Here's how the part is built. I have some questions about the finished solid (model axes, mm). A direction names the side the tool comes from. Round coordinates to 2 decimals unless told otherwise and drop trailing zeros. Order: outer loops, then holes, each group sorted by start corner. A loop starts at its lowest first (then second) coordinate and runs counter-clockwise, first axis right, second up.
Autodesk Inventor part; units mm, degrees
ref_plane "YZ Plane" through (0, 0, 0) normal (1, 0, 0) x (0, 1, 0)
ref_plane "XZ Plane" through (0, 0, 0) normal (0, 1, 0) x (-1, 0, 0)
ref_plane "XY Plane" through (0, 0, 0) normal (0, 0, 1) x (1, 0, 0)
sketch "Sketch1" plane through (0, 0, 0) normal (0, 0, 1) x (1, 0, 0)
  line L0 (0, 40.85) -> (0, 0)
  line L1 (0, 0) -> (-17, 0)
  line L2 (-17, 0) -> (-17, -5)
  line L3 (-17, -5) -> (5, -5)
  line L4 (5, -5) -> (5, 40.85)
  line L5 (5, 40.85) -> (0, 40.85)
  line L6 (-17, 0) -> (-17, 4)
  line L7 (-17, 4) -> (-15, 4)
  line L8 (-15, 4) -> (-15, 0)
  line L9 (-17, -5) -> (-17, -9)
  line L10 (-17, -9) -> (-15, -9)
  line L11 (-15, -9) -> (-15, -5)
  line L12 (-9, 0) -> (-9, 4)
  line L13 (-9, 4) -> (0, 4)
  line L14 (-9, -5) -> (-9, -9)
  line L15 (-9, -9) -> (5, -9)
  line L16 (5, -9) -> (5, -5)
  line L17 (-15, 4) -> (-9, 4)
  line L18 (-15, -9) -> (-9, -9)
  dimension "d0" = 5
  dimension "d1" = 15
  dimension "d2" = 4
  dimension "d3" = 2
  dimension "d4" = 40.85
  dimension "d5" = 6
extrude "Extrusion1" add sketch "Sketch1" along normal blind 25
sketch "Sketch2" plane through (-17, 4, 0) normal (0, 1, 0) x (1, 0, 0)
  circle A0 centre (-1.4373, -213.5) radius 4.5
  line L0 (16.4159, -222.1385) -> (44.0445, -254.6126)
  line L1 (44.0445, -254.6126) -> (38.713, -259.1485)
  line L2 (38.713, -259.1485) -> (11.0845, -226.6745)
  line L3 (11.0845, -226.6745) -> (16.4159, -222.1385)
  line L4 (1.9901, -210.584) -> (-347.6847, 200.416)
  circle A1 centre (-351.112, 197.5) radius 4.5
  point P0 (17, 0)
  point P1 (41.3788, -256.8805)
  dimension "d8" = 7
extrude "Extrusion2" cut sketch "Sketch2" against normal blind 3 contours L0 L1 L2 L3
sketch "Sketch3" plane through (-17, -9, 0) normal (0, -1, 0) x (1, 0, 0)
  line L0 (1.9991, 25) -> (2.3222, 0)
  line L1 (9.3228, 0) -> (8.9997, 25)
  line L2 (22, 225.4393) -> (22, 219.5607) construction
  line L3 (22, 225.4393) -> (-378, 225.4393) construction
  line L4 (-378, 219.5607) -> (-378, 225.4393) construction
  line L5 (22, 219.5607) -> (-378, 219.5607) construction
  circle A0 centre (6.5, 222.5) radius 4.5 construction
  line L6 (-355.6868, -191.4906) -> (9.8625, 219.5094) construction
  line L7 (70.9842, 282.9643) -> (65.7537, 287.6164)
  line L8 (65.7537, 287.6164) -> (-8.4745, 204.1589)
  line L9 (-8.4745, 204.1589) -> (-3.244, 199.5068)
  line L10 (-3.244, 199.5068) -> (70.9842, 282.9643)
  line L11 (2.3222, 0) -> (9.3228, 0)
  line L12 (8.9997, 25) -> (1.9991, 25)
  circle A1 centre (-359.0493, -188.5) radius 4.5
  point P0 (17, 0)
  point P1 (68.369, 285.2903)
  dimension "d38" = 7
extrude "Extrusion3" cut sketch "Sketch3" against normal blind 3 contours L10 L9 L8 L7
chamfer "Chamfer1" distance 7.75 angle 45 1 edges at (5, -9, 12.5)
chamfer "Chamfer3" distance 6 angle 45 1 edges at (0, 4, 12.5)
sketch "Sketch5" plane through (0, 40.85, 0) normal (-1, 0, 0) x (0, 0, 1)
  line L0 (212.5, -7.0607) -> (212.5, -12.9393)
  line L1 (-187.5, -7.0607) -> (212.5, -7.0607)
  line L2 (-187.5, -12.9393) -> (-187.5, -7.0607)
  line L3 (-187.5, -12.9393) -> (212.5, -12.9393)
  line L4 (12.5, -7.0607) -> (12.5, -12.9393) construction
  line L5 (12.5, -10) -> (25, -10) construction
  line L6 (25, -42.1) -> (25, 0)
  line L7 (12.5, -10) -> (0, -10) construction
  line L8 (0, -42.1) -> (0, 0)
  point P0 (0, -40.85)
hole "Hole1" at (0, 30.85, 12.5) direction (1, 0, 0) diameter 3.4 end through all counterbore diameter 6.5 counterbore depth 3.4
fillet "Fillet3" radius 2 6 edges at (-17, 4, 12.5) (-17, -9, 12.5) (5, -1.25, 12.5) (0, 10, 12.5) (5, 40.85, 12.5) (0, 40.85, 12.5)
chamfer "Chamfer4" [suppressed]
properties part number "belt no touchy"
1. If we section it at B-B, the plane z = 12.5: Write out the boundary of the cut face in (x, y).
Evaluation:
outline: (-17, -7) arc R2 ccw to (-15, -9) - (-2.75, -9) - (4.41, -1.84) arc R2 ccw to (5, -0.42) - (5, 29.15) - (3.4, 29.15) - (3.4, 27.6) - (0, 27.6) - (0, 10.83) arc R2 cw to (-0.59, 9.41) - (-6, 4) - (-15, 4) arc R2 ccw to (-17, 2) - close; (0, 34.1) - (3.4, 34.1) - (3.4, 32.55) - (5, 32.55) - (5, 38.85) arc R2 ccw to (3, 40.85) - (2, 40.85) arc R2 ccw to (0, 38.85) - close
2. I'm going to push flat-ended pins straight in: P1, Ø4, axis at y = 23.5, z = 21, coming from the -X side; P2, Ø2.5, axis at x = -12, z = 9, coming from the +Y side; P3, Ø5, axis at x = 1.5, z = 5, coming from the -Y side. Where does each tip first touch, or does it pass through?
Evaluation:
P1: stops at x = 0
P2: stops at y = 4
P3: stops at y = -7.25
3. If we mould it in two halves opening along Z, with no side actions, what happens to faces 4 (the cylindrical face through (-16.43, -8.4, 12.68)), 5 (the flat face through (-4, 5, 0)), 6 (the flat face through (3.4, 32, 14))? For each: released by +Z, released by -Z, zero draft, split by the parting line, or undercut.
Evaluation:
face 4: zero draft
face 5: released by -Z
face 6: undercut
4. If we section it at A-A, the plane y = 30.85: Write out the boundary of the cut face in (x, z).
Evaluation:
outline: (0, 0) - (5, 0) - (5, 10.8) - (3.4, 10.8) - (3.4, 9.25) - (0, 9.25) - close; (0, 15.75) - (3.4, 15.75) - (3.4, 14.2) - (5, 14.2) - (5, 25) - (0, 25) - close
5. If we section it at D-D, the plane x = -5.5: Write out the boundary of the cut face in (y, z).
Evaluation:
outline: (-9, 0) - (4.5, 0) - (4.5, 25) - (-9, 25) - close
6. On a 3-axis mill with a long thin cutter (end or side, diameter ignored), from which of +Z, -Z, +X, -X, +Y, -Y can I reach the whole of each face in a straight line? I mean faces 1 (the cylindrical face through (4.21, 32.36, 13.28)), 2 (the flat face through (0, 25, 12)), 3 (the cylindrical face through (1.7, 32.8, 9.9)). Say none if no direction works.
Evaluation:
face 1: +X, -X
face 2: +Z, -Z, -X, +Y
face 3: -X
7. If we section it at C-C, the plane z = 19.25: Write out the boundary of the cut face in (x, y), and give its area (3 significant figures).
Evaluation:
outline: (-17, -7) arc R2 ccw to (-15, -9) - (-2.75, -9) - (4.41, -1.84) arc R2 ccw to (5, -0.42) - (5, 38.85) arc R2 ccw to (3, 40.85) - (2, 40.85) arc R2 ccw to (0, 38.85) - (0, 10.83) arc R2 cw to (-0.59, 9.41) - (-6, 4) - (-15, 4) arc R2 ccw to (-17, 2) - close
area: 455 mm2
8. I need wall thicknesses on probe 1 along Z at (x, y) = (4.2, 30.85); probe 2 along Z at (x, y) = (1.75, 30.85); probe 3 along Y at (x, z) = (-6.75, 3). Which ranges of each line are inside material? Lowest first, please.
Evaluation:
probe 1: z = 0 to 10.8, 14.2 to 25
probe 2: z = 0 to 9.25, 15.75 to 25
probe 3: y = -9 to 4
